Check sheet for the modelled part. Datum: model origin and axes. Units: mm. A direction names the side the tool comes from. Round coordinates to 2 decimals unless told otherwise and drop trailing zeros. Order: outer loops, then holes, each group sorted by start corner. A loop starts at its lowest first (then second) coordinate and runs counter-clockwise, first axis right, second up.
(1) Sectioned sample at B-B, the plane x = 72. Enter the section's corners in (y, z), and give its area (3 significant figures).
(2) Sectioned sample at C-C, the plane y = 17.5. Enter the section's corners in (x, z), and give its area (3 significant figures).
(3) Thickness scan on probe 1 along Y at (x, z) = (26, 0.3); probe 2 along Y at (x, z) = (65.5, 2.5); probe 3 along X at (y, z) = (10.5, 1.75). Record the ranges inside material, lowest first.
(4) Tool access check on faces 1 (the cylindrical face through (58.996, 22.652, 2.354)), 2 (the flat face through (68, 34.055, 2)), 3 (the flat face through (25, 45.223, 2)). Record the directions out of +Z, -Z, +X, -X, +Y, -Y that give a thin tool (end or side, any length) a straight path to the whole face; none if there is none.
(5) Mould release check, pull along X, two halves, no side actions. Record for faces 4 (the flat face through (51.99, 5.53, 2.35)), 5 (the cylindrical face through (7.79, 35.65, 2.35)), 6 (the flat face through (68, 11.167, 2)): released by +X, released by -X, zero draft, split by the parting line, or undercut.
(6) Depth check by flat-ended pin: pin 1 (10.5 mm diameter, centred on x = 71.96, y = 22.61, fed in from -Z); pin 2 (2.5 mm diameter, centred on x = 63.5, z = 3, fed in from +Y); pin 3 (1.4 mm diameter, centred on x = 73.5, z = 1.5, fed in from -Y). Enter the tip coordinate at first touch or a pass-through.
(7) Sectioned sample at A-A, the plane z = 2.9. Enter the section's corners in (x, y) (3 decimals).
(8) Sectioned sample at D-D, the plane x = 36.5. Enter the section's corners in (y, z).
```python
from build123d import *

# Parameters (mm, degrees)
EXTRUDE1_DEPTH = 4.7752


with BuildPart() as part:
    # Sketch1 → Extrude1 (new body)
    with BuildSketch(Plane.XY):
        with BuildLine():
            Line((0, 42.047652439), (0, 3.175))
            ThreePointArc((0, 3.175), (0.92993597, 0.92993597), (3.175, 0))
            Line((3.175, 0), (47.081976454, 0))
            ThreePointArc((47.081976454, 0), (48.700425311, 0.443471436), (49.866757105, 1.650001072))
            Line((49.866757105, 1.650001072), (54.175007162, 9.517240307))
            ThreePointArc((54.175007162, 9.517240307), (55.341338955, 10.723769944), (56.959787812, 11.167241379))
            Line((56.959787812, 11.167241379), (79.555795926, 11.167241379))
            ThreePointArc((79.555795926, 11.167241379), (81.800859957, 12.097177349), (82.730795926, 14.342241379))
            Line((82.730795926, 14.342241379), (82.730795926, 30.88041106))
            ThreePointArc((82.730795926, 30.88041106), (81.800859957, 33.12547509), (79.555795926, 34.05541106))
            Line((79.555795926, 34.05541106), (56.959787812, 34.05541106))
            ThreePointArc((56.959787812, 34.05541106), (55.341338955, 34.498882496), (54.175007162, 35.705412132))
            Line((54.175007162, 35.705412132), (49.866757105, 43.572651367))
            ThreePointArc((49.866757105, 43.572651367), (48.700425311, 44.779181004), (47.081976454, 45.222652439))
            Line((47.081976454, 45.222652439), (3.175, 45.222652439))
            ThreePointArc((3.175, 45.222652439), (0.92993597, 44.29271647), (0, 42.047652439))
        make_face()
        with BuildLine():
            Line((65.754365641, 24.481484037), (60.865717892, 24.481484037))
            ThreePointArc((60.865717892, 24.481484037), (58.995560075, 22.61132622), (60.865717892, 20.741168403))
            Line((60.865717892, 20.741168403), (65.754365641, 20.741168403))
            ThreePointArc((65.754365641, 20.741168403), (78.445201373, 22.61132622), (65.754365641, 24.481484037))
        make_face(mode=Mode.SUBTRACT)
        with BuildLine():
            Line((10.353425124, 38.271016828), (42.192963273, 38.271016828))
            ThreePointArc((42.192963273, 38.271016828), (44.758567969, 35.705412132), (42.192963273, 33.139807437))
            Line((42.192963273, 33.139807437), (10.353425124, 33.139807437))
            ThreePointArc((10.353425124, 33.139807437), (7.787820428, 35.705412132), (10.353425124, 38.271016828))
        make_face(mode=Mode.SUBTRACT)
        with BuildLine():
            Line((10.353425124, 6.951635611), (42.192963273, 6.951635611))
            ThreePointArc((42.192963273, 6.951635611), (44.758567969, 9.517240307), (42.192963273, 12.082845003))
            Line((42.192963273, 12.082845003), (10.353425124, 12.082845003))
            ThreePointArc((10.353425124, 12.082845003), (7.787820428, 9.517240307), (10.353425124, 6.951635611))
        make_face(mode=Mode.SUBTRACT)
    extrude(amount=EXTRUDE1_DEPTH)


solid = part.part
```
Derived:
1. outline: (11.17, 0) - (16.13, 0) - (16.13, 4.78) - (11.17, 4.78) - close; (29.09, 0) - (34.06, 0) - (34.06, 4.78) - (29.09, 4.78) - close
1. area: 47.4 mm2
2. outline: (0, 0) - (67.97, 0) - (67.97, 4.78) - (0, 4.78) - close; (75.95, 0) - (82.73, 0) - (82.73, 4.78) - (75.95, 4.78) - close
2. area: 357 mm2
3. probe 1: y = 0 to 6.95, 12.08 to 33.14, 38.27 to 45.22
3. probe 2: y = 11.17 to 20.74, 24.48 to 34.06
3. probe 3: x = 0 to 7.98, 44.56 to 55.01
4. face 1: +Z, -Z
4. face 2: +Z, -Z, +X, +Y
4. face 3: +Z, -Z, +X, -X, +Y
5. face 4: released by +X
5. face 5: undercut
5. face 6: zero draft
6. pin 1: passes through
6. pin 2: stops at y = 34.06
6. pin 3: stops at y = 11.17
7. outline: (0, 3.175) arc R3.175 ccw to (3.175, 0) - (47.082, 0) arc R3.175 ccw to (49.867, 1.65) - (54.175, 9.517) arc R3.175 cw to (56.96, 11.167) - (79.556, 11.167) arc R3.175 ccw to (82.731, 14.342) - (82.731, 30.88) arc R3.175 ccw to (79.556, 34.055) - (56.96, 34.055) arc R3.175 cw to (54.175, 35.705) - (49.867, 43.573) arc R3.175 ccw to (47.082, 45.223) - (3.175, 45.223) arc R3.175 ccw to (0, 42.048) - close; hole (10.353, 6.952) - (42.193, 6.952) arc R2.566 ccw to (42.193, 12.083) - (10.353, 12.083) arc R2.566 ccw to start; hole (10.353, 33.14) - (42.193, 33.14) arc R2.566 ccw to (42.193, 38.271) - (10.353, 38.271) arc R2.566 ccw to start; hole (60.866, 20.741) - (65.754, 20.741) arc R6.483 ccw (long way) to (65.754, 24.481) - (60.866, 24.481) arc R1.87 ccw to start
8. outline: (0, 0) - (6.95, 0) - (6.95, 4.78) - (0, 4.78) - close; (12.08, 0) - (33.14, 0) - (33.14, 4.78) - (12.08, 4.78) - close; (38.27, 0) - (45.22, 0) - (45.22, 4.78) - (38.27, 4.78) - close
